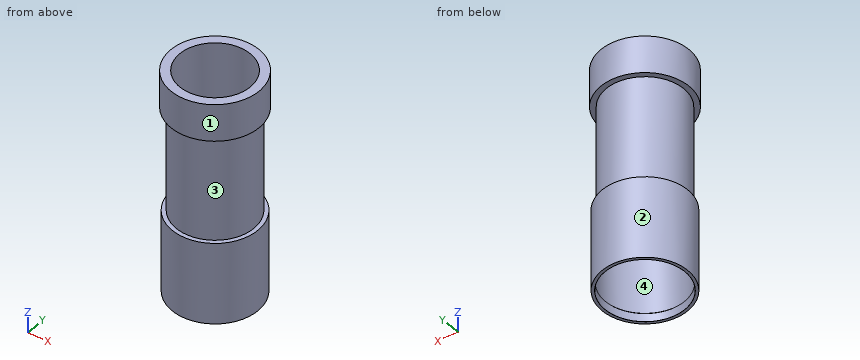
Autodesk Fusion 360 part; units mm, degrees
sketch "Sketch1" plane through (0, 0, 0) normal (1, 0, 0) x (0, 0, -1)
  line L0 (-41.9028, 11) -> (-71.5, 11)
  line L1 (-82, 11) -> (-82, 12.5)
  line L2 (-82, 12.5) -> (-71.5, 12.5)
  line L3 (-71.5, 12.5) -> (-71.5, 11)
  line L4 (-71.5, 11) -> (-41.9028, 11)
  line L5 (-41, 11) -> (-41, 10)
  line L6 (-41, 10) -> (-82, 10)
  line L7 (-82, 10) -> (-82, 11)
  line L8 (-21.273, 11.3453) -> (-41, 11.3453)
  line L9 (-41, 11.3453) -> (-41, 11)
  line L10 (-21.273, 12.1453) -> (-41.9028, 12.1453)
  line L11 (-41.9028, 12.1453) -> (-41.9028, 11)
  line L12 (-20.7884, 12.1453) -> (-21.273, 12.1453)
  line L13 (-20.7884, 12.1453) -> (-18.8, 12.1453)
  line L14 (-18.8, 12.1453) -> (-18.8, 11.3453)
  line L15 (-21.1992, 11.3453) -> (-21.273, 11.3453)
  line L16 (-21.1992, 11.3453) -> (-21.0412, 11.2127)
  line L17 (-18.8, 11.3453) -> (-18.8139, 11.3287)
  line L18 (-21.0412, 11.2127) -> (-18.8139, 11.3287)
  point P0 (-20.7884, 10.9915)
  dimension "d1" = 1.5
  dimension "d2" = 10.5
  dimension "d3" = 0.8
  dimension "d4" = 0.6
revolve "Revolve1" add sketch "Sketch1" angle 360 about axis through (0, 0, 1.75) along (0, 0, 1)
Geometry: final body of the model. Coordinates: model frame, mm. Face numbers are marked on the shaded views. A direction names the side the tool comes from. Round coordinates to 2 decimals unless told otherwise and drop trailing zeros. Order: outer loops, then holes, each group sorted by start corner. A loop starts at its lowest first (then second) coordinate and runs counter-clockwise, first axis right, second up.
Q1. Section C-C, the plane z = 63. Output: boundary loops of the cut face in (x, y).
Result sheet:
outline: circle Ø22 at (0, 0); hole circle Ø20 at (0, 0)
Q2. Pin query (flat end, axial travel): pin 1 (3 mm diameter, centred on x = 6, z = 69.5, fed in from +Y); pin 2 (1 mm diameter, centred on x = -2, y = -8.5, fed in from -Z); pin 3 (5 mm diameter, centred on y = 3, z = 68, fed in from +X); pin 4 (6 mm diameter, centred on y = -7.5, z = 45.5, fed in from +X). Return the tip coordinate at first contact, or that it passes through.
Result sheet:
pin 1: stops at y = 10.04
pin 2: passes through
pin 3: stops at x = 10.99
pin 4: stops at x = 10.04
Q3. Access query for the marked faces 1 and 2. Directions: +Z, -Z, +X, -X, +Y, -Y. A direction counts if a zero-diameter tool reaches every point of the face in a straight line with its end or side. Return the directions, or none.
Result sheet:
face 1: +Z, -Z
face 2: -Z
Q4. Mould query, pull axis Y, two halves, no side actions, for the marked faces 3 and 4. Classes: released by +Y, released by -Y, zero draft, split by the parting line, or undercut.
Result sheet:
face 3: split by the parting line
face 4: undercut
Q5. Section D-D, the plane z = 32. Output: boundary loops of the cut face in (x, y), and give its area (3 significant figures).
Result sheet:
outline: circle Ø24.29 at (0, 0); hole circle Ø22.69 at (0, 0)
area: 59.0 mm2
Q6. Material intervals for probe 1 along Z at (x, y) = (6.5, -9.75); probe 2 along X at (y, z) = (0, 31); probe 3 along Z at (x, y) = (8.5, -7.25), sorted ascending.
Result sheet:
probe 1: z = 18.8 to 41.9, 71.5 to 82
probe 2: x = -12.15 to -11.35, 11.35 to 12.15
probe 3: z = 41 to 41.9, 71.5 to 82
